Could you check a few things on this model? Use its own coordinates, in mm. A direction names the side the tool comes from. Coordinates: 2 decimals unless noted, no trailing zeros. Order: outer loops, then holes, each group sorted by start corner. A loop starts at its lowest first (then second) coordinate and runs counter-clockwise, first axis right, second up. Notation, with made-up numbers: (80.25, 15.5) - (117.25, 15.5) arc R23 ccw to (117.25, 43.5) - close; hole circle Ø5 at (18.25, 74). An arc over 180 degrees is marked (long way). One line per item, written item: value. Start each with the question number.
from build123d import *

# Parameters (mm, degrees)
F0_R         = 7
F1_DEPTH     = 560
F2_R         = 7
F2_R_2       = 6
F3_DEPTH     = 40
F4_R         = 2.75
F5_DEPTH     = 560.001
F6_R         = 1.75
F7_DEPTH     = 10
F8_R         = 13
F8_R_2       = 7
F9_DEPTH     = 70
F10_S5_R     = 7
F10_T6_DEPTH = 22


# Not quite as in the source:
# - a fillet or chamfer that OpenCascade refuses, or shapes differently, is made with other operations: its cross-section is extruded or revolved along the edge and cut away or added


with BuildPart() as f1:
    # F0 (on Front) → F1 (new body)
    with BuildSketch(Plane.XZ):
        Circle(F0_R)
    extrude(amount=-F1_DEPTH)

    # F2 (on face) → F3 (cut)
    with BuildSketch(Plane.XZ):
        Circle(F2_R)
        Circle(F2_R_2, mode=Mode.SUBTRACT)
    extrude(amount=-F3_DEPTH, mode=Mode.SUBTRACT)

    # F4 (on face) → F5 (cut, through all)
    with BuildSketch(Plane.XZ):
        Circle(F4_R)
    extrude(amount=-F5_DEPTH, mode=Mode.SUBTRACT)

    # F6 (on Top) → F7 (cut)
    with BuildSketch(Plane.XY):
        with Locations((0, 8)):
            Circle(F6_R)
    extrude(amount=-F7_DEPTH, mode=Mode.SUBTRACT)

    # F8 (on face) → F9 (join)
    with BuildSketch(Plane(origin=(0, 560, 0), x_dir=(-1, 0, 0), z_dir=(0, 1, 0))):
        Circle(F8_R)
        Circle(F8_R_2, mode=Mode.SUBTRACT)
    extrude(amount=-F9_DEPTH)

    # F10: chamfer of 20 x 8 on 1 edges, made by hand


with BuildPart() as f10_tool2:
    # F10_s3 → F10_t4 (revolve)
    with BuildSketch(Plane.XY):
        Polygon((-5, 490), (-13, 510), (-13, 490), align=None)
    revolve(axis=Axis((0, 490, 0), (0, 1, 0)))

    # F10_s5 → F10_t6 (cut, symmetric)
    with BuildSketch(Plane.XZ.offset(-500)):
        Circle(F10_S5_R)
    extrude(amount=F10_T6_DEPTH, both=True, mode=Mode.SUBTRACT)


with BuildPart() as f1_1:
    add(f1.part)

    # F10_t1: cut F10_tool2
    add(f10_tool2.part, mode=Mode.SUBTRACT)


solid = f1_1.part
Q1. If I drill on L1, parallel to Z at x = 0, y = 415; L2, parallel to Y at x = 0, z = -3.25; L3, parallel to X at y = 8, z = -3, over which ranges is the centre line in solid material (lowest first)?
Q2. I want a section at B-B on y = 502.5. Please give me the cut outline in (x, z).
Q3. Which directions (+Z, -Z, +X, -X, +Y, -Y) give clear straight access to the entire face, cutting with the end or side of a thin tool? Please do faces 1 (the cylindrical face through (10.316, 535.35, -7.91)), 2 (the cylindrical face through (6.466, 264.315, -2.681)).
Q4. I want a section at A-A on y = 203.5. Please give me the cut outline in (x, z).
Q5. I'm going to push flat-ended pins straight in: pin 1 (12 mm diameter, centred on x = 10, y = 389.5, fed in from -Z); pin 2 (4 mm diameter, centred on x = 3.5, y = 330, fed in from +Z); pin 3 (3 mm diameter, centred on x = -10, y = 91.5, fed in from -Z); pin 4 (4 mm diameter, centred on x = 0, y = 8, fed in from -Z). Where does each tip first touch, or does it pass through?
Values follow:
1. L1: z = -7 to -2.75, 2.75 to 7
1. L2: y = 0 to 6.25, 9.75 to 560
1. L3: x = -5.2 to -1.75, 1.75 to 5.2
2. outline: circle Ø20 at (0, 0); hole circle Ø5.5 at (0, 0)
3. face 1: +Y, -Y
3. face 2: -Y
4. outline: circle Ø14 at (0, 0); hole circle Ø5.5 at (0, 0)
5. pin 1: stops at z = -5.74
5. pin 2: stops at z = 6.84
5. pin 3: passes through
5. pin 4: stops at z = -6
